```python
from build123d import *

# Parameters (mm, degrees)
SWEEP1_PROFILE_R        = 11
CUT_EXTRUDE1_DEPTH      = 139.5211963076765
CUT_EXTRUDE1_DEPTH_BACK = 139.5211963076765
BOSS_EXTRUDE1_DEPTH     = 11
BOSS_EXTRUDE4_DEPTH     = 11
SHELL1_START            = -11
SHELL1_DEPTH            = 11
SHELL1_START_2          = -113.150665538
SHELL1_2_DEPTH          = 47.855548818
SHELL1_START_3          = 20.420083618
SHELL1_3_DEPTH          = 73.048431747
FILLET1_R               = 6.5
BOSS_EXTRUDE2_DEPTH     = 3
CUT_EXTRUDE2_DEPTH      = 13.000000000000002
SKETCH21_R              = 2.499999999999935
SKETCH21_R_2            = 2.499999999999995
BOSS_EXTRUDE3_DEPTH     = 2
SKETCH22_R              = 1.4999999999999973
SKETCH22_R_2            = 1.5000000000000042
CUT_EXTRUDE3_DEPTH      = 13.000000000000002
FILLET2_R               = 3.75
CUT_EXTRUDE4_DEPTH      = 3
FILLET3_R               = 20
CUT_EXTRUDE5_DEPTH      = 3
FILLET4_R               = 1
CUT_EXTRUDE6_DEPTH      = 158.49217492446147
CUT_EXTRUDE7_DEPTH      = 5.1


with BuildPart() as part:
    # Sweep1: sweep along a path in Sketch6
    with BuildLine(Plane(origin=(0, 0, 0), x_dir=(0, 0, -1), z_dir=(1, 0, 0))) as sweep1_path:
        Line((17.67333262983066, 12.262734264551655), (84.99999999999999, 32.11621443102775))
        Line((84.99999999999999, 32.11621443102775), (127.09238599616681, 16.202979651458282))
    # Sweep1 profile (on start of the path) → Sweep1 (sweep)
    with BuildSketch(Plane(origin=(0, 12.262734264551655, -17.67333262983066), x_dir=(0, -0.9591665787285488, -0.28284178306991825), z_dir=(0, 0.28284178306991825, -0.9591665787285488))):
        Circle(SWEEP1_PROFILE_R)
    sweep(path=sweep1_path.line, transition=Transition.RIGHT)

    # Sketch13 → Cut-Extrude1 (cut, two sides: drawn at the far end of the back side and taken through both)
    with BuildSketch(Plane(origin=(0, 0, 0), x_dir=(1, 0, 0), z_dir=(0, 1, 0)).offset(-CUT_EXTRUDE1_DEPTH_BACK)):
        Polygon((-1.735e-14, 141.7207506217034), (-10.000000000000018, 141.7207506217034), (-10, -2.41e-15), (0, -1.18e-15), align=None)
    extrude(amount=CUT_EXTRUDE1_DEPTH + CUT_EXTRUDE1_DEPTH_BACK, mode=Mode.SUBTRACT)


with BuildPart() as cut_extrude1_piece_1:
    # of the separate pieces the step leaves, piece 1, a body of its own (cut_extrude1_pieces)
    add(part.part.solids().sort_by_distance((0, 22.813566631, -14.562073016))[0])



with BuildPart() as cut_extrude1_piece_2:
    # of the separate pieces the step leaves, piece 2, a body of its own (cut_extrude1_pieces)
    add(part.part.solids().sort_by_distance((-10, 7.867280813, -18.96947651))[0])


with BuildPart() as cut_extrude1_piece_1_1:
    add(cut_extrude1_piece_1.part)

    add(cut_extrude1_piece_2.part)  # Boss-Extrude1 merges Cut-Extrude1 piece 2
    # Sketch17 → Boss-Extrude1 (add)
    with BuildSketch(Plane(origin=(0, 0, 0), x_dir=(0, 0, -1), z_dir=(1, 0, 0))):
        Polygon((14.562073016061587, 22.813566630565735), (85.43326002077312, 43.71226488094253), (130.98228783117273, 26.4922295616324), (123.20248416116098, 5.91372974128417), (84.56673997922682, 20.52016398111302), (20.78459224359979, 1.7119018985376593), align=None)
    extrude(amount=-BOSS_EXTRUDE1_DEPTH)

    # Sketch24 → Boss-Extrude4 (add)
    with BuildSketch(Plane(origin=(0, 0, 0), x_dir=(0, 0, -1), z_dir=(1, 0, 0))):
        Polygon((127.09238599616687, 16.20297965145829), (84.99999999999997, 32.11621443102777), (17.673332629830696, 12.2627342645517), (14.5620730160616, 22.813566630565738), (85.43326002077312, 43.71226488094253), (130.98228783117273, 26.4922295616324), align=None)
    extrude(amount=BOSS_EXTRUDE4_DEPTH)

    # Shell1: read off the stored shape, not the designer's step
    # Shell1 outline → Shell1 (cut)
    with BuildSketch(Plane.YZ.offset(SHELL1_START)):
        Polygon((4.109818345, -20.077487786), (23.155629992, -84.665208166), (8.25219563, -124.08655276), (24.153763673, -130.098219232), (41.07679887, -85.334791834), (20.415650184, -15.269177474), align=None)
    extrude(amount=SHELL1_DEPTH, mode=Mode.SUBTRACT)

    # Shell1 2 outline → Shell1 2 (cut)
    with BuildSketch(Plane(origin=(0, 0, 0), x_dir=(1, 0, 0), z_dir=(0, 0.353627439545988, 0.935386355470374)).offset(SHELL1_START_2)):
        with BuildLine():
            ThreePointArc((0, 51.59940113), (6.01040764, 54.088993489), (8.5, 60.09940113))
            Line((8.5, 60.09940113), (8.5, 68.59940113))
            Line((8.5, 68.59940113), (0, 68.59940113))
            Line((0, 68.59940113), (0, 51.59940113))
        make_face()
    extrude(amount=SHELL1_2_DEPTH, mode=Mode.SUBTRACT)

    # Shell1 3 outline → Shell1 3 (cut)
    with BuildSketch(Plane(origin=(0, 0, 0), x_dir=(1, 0, 0), z_dir=(0, 0.2828417830699179, -0.9591665787285488)).offset(SHELL1_START_3)):
        with BuildLine():
            Line((8.5, -15.263247957), (8.5, -6.763247957))
            ThreePointArc((8.5, -6.763247957), (6.01040764, -0.752840317), (0, 1.736752043))
            Line((0, 1.736752043), (0, -15.263247957))
            Line((0, -15.263247957), (8.5, -15.263247957))
        make_face()
    extrude(amount=SHELL1_3_DEPTH, mode=Mode.SUBTRACT)

    # Fillet1
    fillet1_edges = [cut_extrude1_piece_1_1.edges().sort_by_distance(p)[0] for p in [
        (7.881335387835811, 24.026781093815067, -84.69775674305134),
        (6.090122796410721, 25.865288676138242, -84.76644839135132),
        (-5.5, 23.155629992, -84.665208166),
        (-5.5, 20.52016398111302, -84.56673997922682),
    ]]
    fillet(fillet1_edges, radius=FILLET1_R)

    # Sketch19 → Boss-Extrude2 (add)
    with BuildSketch(Plane(origin=(-11, 0, 0), x_dir=(0, 0, -1), z_dir=(1, 0, 0))):
        Polygon((23.326841994418306, 17.839501416273155), (61.69350514356026, 29.153172739069877), (63.814818516584644, 21.959423398605768), (25.44815536744269, 10.645752075809039), align=None)
        with BuildLine():
            Line((82.27394375020691, 30.863769892150234), (86.9487114072542, 20.688724856427108))
            Line((86.9487114072542, 20.688724856427108), (97.3098397387939, 16.771649028602706))
            Line((97.3098397387939, 16.771649028602706), (109.44211139391379, 26.082981771484846))
            Line((109.44211139391379, 26.082981771484846), (86.06088152658778, 34.92237140237257))
            ThreePointArc((86.06088152658778, 34.92237140237257), (82.80654161714303, 34.162852377504095), (82.27394375020691, 30.863769892150234))
        make_face()
    extrude(amount=-BOSS_EXTRUDE2_DEPTH)


with BuildPart() as boss_extrude2_piece_1:
    # of the separate pieces the step leaves, piece 1, a body of its own (boss_extrude2_pieces)
    add(cut_extrude1_piece_1_1.part.solids().sort_by_distance((-1e-09, 22.538001125, -82.570719291))[0])

    # Sketch20 → Cut-Extrude2 (cut)
    with BuildSketch(Plane(origin=(0, 45.92690987835062, -17.362895504685262), x_dir=(1, 0, 0), z_dir=(0, -0.9353863554703739, 0.3536274395459883))):
        Polygon((-11.00000000000001, -75.16519001409192), (3.999999999999988, -75.16519001409192), (3.9999999999999916, -85.1651900140919), (-11.00000000000001, -85.1651900140919), align=None)
    extrude(amount=-CUT_EXTRUDE2_DEPTH, mode=Mode.SUBTRACT)



with BuildPart() as boss_extrude2_piece_2:
    # of the separate pieces the step leaves, piece 2, a body of its own (boss_extrude2_pieces)
    add(cut_extrude1_piece_1_1.part.solids().sort_by_distance((-11, 17.839501416, -23.326841994))[0])


with BuildPart() as boss_extrude2_piece_1_1:
    add(boss_extrude2_piece_1.part)

    add(boss_extrude2_piece_2.part)  # Boss-Extrude3 merges Boss-Extrude2 piece 2
    # Sketch21 → Boss-Extrude3 (add)
    # profile 1 of 2: a face of its own
    with BuildSketch(Plane.ZY.offset(11)):
        with BuildLine():
            Line((-59.92574399937327, 35.14796385612329), (-14.844914799131477, 21.85440005183715))
            Line((-14.844914799131477, 21.85440005183715), (-15.269177473736278, 20.4156501837443))
            Line((-15.269177473736278, 20.4156501837443), (-7.49992818603503, 18.124631740877966))
            ThreePointArc((-7.49992818603503, 18.124631740877966), (-3.391731998282636, 14.806195907785265), (-2.833287095990472, 9.554774044468546))
            Line((-2.833287095990472, 9.554774044468546), (-3.738380801814209, 6.4854409925371845))
            ThreePointArc((-3.738380801814209, 6.4854409925371845), (-7.056816634906908, 2.377244804784792), (-12.308238498223627, 1.8187999024926287))
            Line((-12.308238498223627, 1.8187999024926287), (-20.07748778592488, 4.1098183453589545))
            Line((-20.07748778592488, 4.1098183453589545), (-20.501750460529845, 2.6710684772661613))
            Line((-20.501750460529845, 2.6710684772661613), (-65.58257966077163, 15.964632281552323))
            Line((-65.58257966077163, 15.964632281552323), (-59.92574399937327, 35.14796385612329))
        make_face()
        with Locations((-10.000000000002185, 9.999999999992289)):
            Circle(SKETCH21_R, mode=Mode.SUBTRACT)
    # profile 2 of 2: a face of its own
    with BuildSketch(Plane.ZY.offset(11)):
        with BuildLine():
            Line((-97.3098397387939, 16.771649028602706), (-97.8402808981129, 18.1747285618083))
            Line((-97.8402808981129, 18.1747285618083), (-140.4938987075619, 2.049317318511217))
            ThreePointArc((-140.4938987075619, 2.049317318511217), (-145.77235119424373, 2.21433744231316), (-149.3880938931748, 6.0634538383894725))
            Line((-149.3880938931748, 6.0634538383894725), (-150.519701699722, 9.056690175894678))
            ThreePointArc((-150.519701699722, 9.056690175894678), (-150.35468157592004, 14.33514266257649), (-146.50556517984373, 17.95088536150758))
            Line((-146.50556517984373, 17.95088536150758), (-103.85194737039468, 34.07629660480464))
            Line((-103.85194737039468, 34.07629660480464), (-104.38238852971367, 35.479376138010196))
            Line((-104.38238852971367, 35.479376138010196), (-94.02126019817398, 39.39645196583461))
            Line((-94.02126019817398, 39.39645196583461), (-86.9487114072542, 20.688724856427108))
            Line((-86.9487114072542, 20.688724856427108), (-97.3098397387939, 16.771649028602706))
        make_face()
        with Locations((-143.4999999999837, 10.000000000006171)):
            Circle(SKETCH21_R_2, mode=Mode.SUBTRACT)
    extrude(amount=-BOSS_EXTRUDE3_DEPTH)

    # Sketch22 → Cut-Extrude3 (cut)
    with BuildSketch(Plane.ZY.offset(13.999999999999998)):
        with Locations((-95.66554996848392, 28.084050497218655)):
            Circle(SKETCH22_R)
        with Locations((-43.57083025550148, 19.89946240743944)):
            Circle(SKETCH22_R_2)
    extrude(amount=-CUT_EXTRUDE3_DEPTH, mode=Mode.SUBTRACT)

    # Fillet2
    fillet2_edges = [boss_extrude2_piece_1_1.edges().sort_by_distance(p)[0] for p in [
        (-12.5, 10.645752075809039, -25.44815536744269),
        (-12.5, 17.839501416273155, -23.326841994418306),
        (-12.5, 21.959423398605768, -63.814818516584644),
        (-12.5, 29.153172739069877, -61.69350514356026),
        (-12.5, 26.082981771484846, -109.44211139391379),
    ]]
    fillet(fillet2_edges, radius=FILLET2_R - 0.0001)  # a hair under: the kernel refuses the full size

    # Sketch23 → Cut-Extrude4 (cut)
    with BuildSketch(Plane(origin=(0, 17.03791376961812, 5.024188725151693), x_dir=(1, 0, 0), z_dir=(0, 0.9591665787285488, 0.28284178306991814))):
        Polygon((-11, 23.42008361798458), (8, 23.42008361798471), (8, 28.420083617984712), (-11, 28.420083617984712), align=None)
    extrude(amount=-CUT_EXTRUDE4_DEPTH, mode=Mode.SUBTRACT)

    # Fillet3
    fillet3_edges = [boss_extrude2_piece_1_1.edges().sort_by_distance(p)[0] for p in [
        (0, 43.71226488094253, -85.43326002077312),
        (-5.5, 41.07679887, -85.334791834),
    ]]
    fillet(fillet3_edges, radius=FILLET3_R)

    # Sketch25 → Cut-Extrude5 (cut)
    with BuildSketch(Plane(origin=(0, 66.50540969869883, -25.142699174696986), x_dir=(1, 0, 0), z_dir=(0, 0.9353863554703739, -0.3536274395459882))):
        Polygon((-11, 101.17418781590268), (8, 101.17418781590271), (8, 106.17418781590271), (-11, 106.17418781590268), align=None)
    extrude(amount=-CUT_EXTRUDE5_DEPTH, mode=Mode.SUBTRACT)

    # Fillet4
    fillet4_edges = [boss_extrude2_piece_1_1.edges().sort_by_distance(p)[0] for p in [
        (-4.5, 22.678384448496875, -22.942510103507807),
        (-1.5, 23.66209197977548, -17.439572752247173),
        (8, 24.36919643745029, -19.837489199068607),
        (-1.5, 25.076300895125087, -22.235405645889983),
        (-4.5, 28.388974824561164, -118.89558538463223),
        (-1.5, 30.72744071321624, -119.77965398348931),
        (8, 29.84337211435127, -122.11811987216527),
        (-1.5, 28.959303515486297, -124.45658576084118),
    ]]
    fillet(fillet4_edges, radius=FILLET4_R)

    # Sketch26 → Cut-Extrude6 (cut, through all)
    with BuildSketch(Plane(origin=(0, 0, 0), x_dir=(0, 0, -1), z_dir=(1, 0, 0))):
        Polygon((-14.446633314427679, 64.99999999999999), (165.5533666855723, 65.00000000000001), (165.55336668557234, -24.99999999999997), (-14.446633314427677, -25.000000000000004), align=None)
    extrude(amount=CUT_EXTRUDE6_DEPTH, mode=Mode.SUBTRACT)

    # Sketch27 → Cut-Extrude7 (cut)
    with BuildSketch(Plane(origin=(0, 0, 0), x_dir=(0, 0, -1), z_dir=(1, 0, 0))):
        Polygon((34.45250904830736, 26.07248584514273), (34.09895681946996, 27.271444068553414), (48.486455500398186, 31.514070814602224), (48.840007729235595, 30.315112591191493), align=None)
        Polygon((58.44415093506696, 15.423489668155758), (58.79770316390435, 14.224531444745072), (73.1852018448326, 18.46715819079385), (72.8316496159952, 19.66611641420453), align=None)
        Polygon((98.3170855642761, 36.16877849455206), (98.75911986370858, 37.33801143889003), (112.78991519576418, 32.03359984570021), (112.34788089633173, 30.864366901362228), align=None)
    extrude(amount=-CUT_EXTRUDE7_DEPTH, mode=Mode.SUBTRACT)


solid = boss_extrude2_piece_1_1.part
```
Verification items for the finished model (mm, model axes). A direction names the side the tool comes from. Coordinates: 2 decimals unless noted, no trailing zeros. Loops run counter-clockwise (first coordinate to the right, second up) from the corner with the lowest first, then second, coordinate; pieces in that order, holes last. Notation, with made-up numbers: (70.25, -5) - (102.25, -5) arc R33 ccw to (102.25, 26) - close; hole circle Ø8 at (86.25, -7.5). An arc over 180 degrees is marked (long way). Return JSON: item names as keys, results as strings.
1. Section check C-C, the plane z = -10. Record the boundary of the cut face in (x, y).
Established:
{"outline": "(-11, 1.55) - (-9, 1.55) - (-9, 7.5) - (-11, 7.5) - close; (-11, 12.5) - (-9, 12.5) - (-9, 18.86) - (-11, 18.86) - close"}
2. Section check B-B, the plane z = -107.5. Record the boundary of the cut face in (x, y).
Established:
{"outline": "(-11, 11.85) - (0, 11.85) - (0, 14.52) - (-9, 14.52) - (-9, 32.7) - (-5.1, 32.7) - (-5.1, 34.03) - (0, 34.03) - (0, 35.37) - (-11, 35.37) - close"}
3. Tool access check on faces 1 (the flat face through (-5.42, 21.6, -14.92)), 2 (the cylindrical face through (-5.423, 39.982, -85.203)), 3 (the flat face through (-9, 20, -119)), 4 (the cylindrical face through (-12.52, 22.74, -62.47)). Record the directions out of +Z, -Z, +X, -X, +Y, -Y that give a thin tool (end or side, any length) a straight path to the whole face; none if there is none.
Established:
{"face 1": "+Z, +X, -X", "face 2": "+X, -X", "face 3": "+X", "face 4": "-X"}
4. Go/stop test with flat-tipped pins: pin 1 (2 mm diameter, centred on x = -6.5, z = -21, fed in from +Y); pin 2 (20.5 mm diameter, centred on y = 32, z = -95, fed in from -X); pin 3 (6.5 mm diameter, centred on y = 10, z = -10, fed in from +X); pin 4 (2.5 mm diameter, centred on y = 28.5, z = -44.5, fed in from +X). Record where each tip stops, or that it passes through.
Established:
{"pin 1": "stops at y = 4.68", "pin 2": "stops at x = -14", "pin 3": "stops at x = -9", "pin 4": "stops at x = -5.1"}
5. Mould release check, pull along Z, two halves, no side actions. Record for faces 5 (the cylindrical face through (-12.521, 25.45, -105.533)), 6 (the flat face through (-12.48, 23.43, -42.29)), 7 (the flat face through (-2.514, 16.316, -65.891)): +Z half, -Z half, draft (parallel to the pull), parting line (faces both ways), or undercut.
Established:
{"face 5": "-Z half", "face 6": "+Z half", "face 7": "undercut"}
6. Section check A-A, the plane z = -143.5. Record the boundary of the cut face in (x, y), then the cut area to 3 significant figures.
Established:
{"outline": "(-11, 1.63) - (-9, 1.63) - (-9, 7.5) - (-11, 7.5) - close; (-11, 12.5) - (-9, 12.5) - (-9, 19.09) - (-11, 19.09) - close", "area": "24.9 mm2"}
7. Section check D-D, the plane z = -54.5. Record the boundary of the cut face in (x, y), then the cut area to 3 significant figures.
Established:
{"outline": "(-14, 19.21) - (-11, 19.21) - (-11, 11.65) - (0, 11.65) - (0, 14.26) - (-9, 14.26) - (-9, 31.98) - (0, 31.98) - (0, 34.59) - (-11, 34.59) - (-11, 27.03) - (-14, 27.03) - close", "area": "116 mm2"}
8. Thickness scan on L1, parallel to X at y = 19, z = -139.5; L2, parallel to X at y = 16, z = -33.5; L3, parallel to Y at x = -11.5, z = -43.5. Record the ranges inside material, lowest first.
Established:
{"L1": "x = -11 to -9", "L2": "x = -14 to -9", "L3": "y = 15.97 to 18.4, 21.4 to 23.79"}
